Autodesk Inventor part; units mm, degrees
ref_plane "YZ Plane" through (0, 0, 0) normal (1, 0, 0) x (0, 1, 0)
ref_plane "XZ Plane" through (0, 0, 0) normal (0, 1, 0) x (-1, 0, 0)
ref_plane "XY Plane" through (0, 0, 0) normal (0, 0, 1) x (1, 0, 0)
sketch "Sketch1" plane through (0, 0, 0) normal (0, 1, 0) x (-1, 0, 0)
  line L0 (0, 0) -> (8, 0)
  line L1 (8, 0) -> (8, -20)
  line L2 (8, -20) -> (0, -20)
  line L3 (0, -20) -> (0, 0)
  dimension "d0" = 8
  dimension "d1" = 20
extrude "Extrusion1" add sketch "Sketch1" along normal blind 3.8
sketch "Sketch2" plane through (0, 0, 0) normal (1, 0, 0) x (0, 0, -1)
  line L0 (20, 3.8) -> (0, 3.8)
  line L1 (0, 3.8) -> (0, 6.8)
  line L2 (0, 6.8) -> (3, 6.8)
  line L3 (3, 6.8) -> (3, -3)
  line L4 (3, -3) -> (0, -3)
  line L5 (0, -3) -> (0, 6.8)
  line L6 (0, 3.8) -> (20, 3.8)
  line L7 (10, 3.8) -> (10, 4.6084)
  line L8 (20, 6.8) -> (17, 6.8)
  line L9 (17, 6.8) -> (17, -3)
  line L10 (17, -3) -> (20, -3)
  line L11 (20, -3) -> (20, 6.8)
  point P0 (0, 0)
  point P1 (0, 3.8)
  dimension "d4" = 3
  dimension "d5" = 3
  dimension "d6" = 9.8
extrude "Extrusion2" add sketch "Sketch2" against normal blind 8
properties part number "cable_jig_lock"
CAD build for the part. Positions are in the model's coordinates, mm. A direction names the side the tool comes from. Round coordinates to 2 decimals unless told otherwise and drop trailing zeros. Order: outer loops, then holes, each group sorted by start corner. A loop starts at its lowest first (then second) coordinate and runs counter-clockwise, first axis right, second up. Notation, with made-up numbers: (29, 76.5) - (58, 76.5) arc R21 cw to (58, 97.5) - close; hole circle Ø9 at (72.25, 85.25). An arc over 180 degrees is marked (long way). Answer in a Markdown table with one row per item. Add a question column.
(1) Band-saw the part on B-B on x = -4.5. List the corners of the cut face in (y, z), and give its area (3 significant figures).
(2) Probe L1, parallel to Z at x = -4, y = 5.5; L2, parallel to Y at x = -0.75, z = -7.75. List the from-to ranges inside material, lowest first. Write a range as [from, to].
(3) Drop flat-ended pins along their axis: pin 1 Ø4 at (x, z) = (-3, -7) entering from +Y; pin 2 Ø2.5 at (x, z) = (-6, -10.5) entering from -Y. Give the stop position or say it passes through.
(4) Mould opens along Z. For faces 1 (the face through (-4, -3, -18)), 2 (the face through (-4, 2, 0)), 3 (the face through (-4, 0, -10)) say: +Z half, -Z half, draft (parallel to the pull), parting line (faces both ways), or undercut.
(5) Band-saw the part on C-C on z = -13.5. List the corners of the cut face in (x, y).
(6) Band-saw the part on A-A on y = 4. List the corners of the cut face in (x, z), and give its area (3 significant figures).
(7) 3-axis set-ups, long thin cutter, end or side, ignore diameter. For faces 4 (the face through (-4, 5, -3)), 5 (the face through (-4, 6.8, -1)), 6 (the face through (-4, -1, -17)): which of +Z, -Z, +X, -X, +Y, -Y reach the whole face in a straight line?
Data:
| question | item | result |
|---|---|---|
| 1 | outline | (-3, -20) - (6.8, -20) - (6.8, -17) - (3.8, -17) - (3.8, -3) - (6.8, -3) - (6.8, 0) - (-3, 0) - (-3, -3) - (0, -3) - (0, -17) - (-3, -17) - close |
| 1 | area | 112 mm^2 |
| 2 | L1 | z = [-20, -17], [-3, 0] |
| 2 | L2 | y = [0, 3.8] |
| 3 | pin 1 | stops at y = 3.8 |
| 3 | pin 2 | stops at y = 0 |
| 4 | face 1 | draft |
| 4 | face 2 | +Z half |
| 4 | face 3 | undercut |
| 5 | outline | (-8, 0) - (0, 0) - (0, 3.8) - (-8, 3.8) - close |
| 6 | outline | (-8, -20) - (0, -20) - (0, -17) - (-8, -17) - close; (-8, -3) - (0, -3) - (0, 0) - (-8, 0) - close |
| 6 | area | 48.0 mm^2 |
| 7 | face 4 | +X, -X, +Y |
| 7 | face 5 | +Z, -Z, +X, -X, +Y |
| 7 | face 6 | +X, -X, -Y |
